from build123d import *

# Parameters (mm, degrees)
BOSS_EXTRUDE1_DEPTH      = 50.8
BOSS_EXTRUDE1_DEPTH_BACK = 38.1
SKETCH1_W                = 381
SKETCH1_H                = 12.7
SKETCH3_W                = 12.7
SKETCH3_H                = 44.45
CUT_EXTRUDE1_DEPTH       = 2664.230012597
CAVITY1_START            = 52.3
CAVITY1_OUTLINE_R        = 12.7
CAVITY1_DEPTH            = 12.7


# Read off the part's stored shape, not the designer's step: Cavity1
with BuildPart() as part:
    # Sketch1 → Boss-Extrude1 (new, two sides: drawn at the far end of the back side and taken through both)
    with BuildSketch(Plane.XY.offset(287.7).offset(-BOSS_EXTRUDE1_DEPTH_BACK)):
        with Locations((2451.1, 58.65)):
            Rectangle(SKETCH1_W, SKETCH1_H)
    extrude(amount=BOSS_EXTRUDE1_DEPTH + BOSS_EXTRUDE1_DEPTH_BACK)

    # Sketch3 → Cut-Extrude1 (cut, through all)
    with BuildSketch(Plane(origin=(0, 65, 0), x_dir=(1, 0, 0), z_dir=(0, 1, 0))):
        with Locations((2470.15, -271.825)):
            Rectangle(SKETCH3_W, SKETCH3_H)
    extrude(amount=-CUT_EXTRUDE1_DEPTH, mode=Mode.SUBTRACT)

    # Cavity1 outline → Cavity1 (cut)
    with BuildSketch(Plane(origin=(0, 0, 0), x_dir=(1, 0, 0), z_dir=(0, 1, 0)).offset(CAVITY1_START)):
        with Locations((2300, -275)):
            Circle(CAVITY1_OUTLINE_R)
        with Locations((2600, -275)):
            Circle(CAVITY1_OUTLINE_R)
    extrude(amount=CAVITY1_DEPTH, mode=Mode.SUBTRACT)


solid = part.part
Can you work these out from the model? Positions are in its coordinate system, mm. A direction names the side the tool comes from. Give positions to 0.01 mm unless a question says otherwise; leave off trailing zeros. Order: outer loops, then holes, each group sorted by start corner. A loop starts at its lowest first (then second) coordinate and runs counter-clockwise, first axis right, second up. Notation, with made-up numbers: M 20.25,88.25 L 43.25,88.25 A26 ccw 43.25,108.25 Z; hole C 33,-9 d5. An arc over 180 degrees is marked long. One line per item, written item: value.
Item 1: If we section it at C-C on y = 60.5: Write out the boundary of the cut face in (x, z).
Verdict:
outline: M 2260.6,249.6 L 2463.8,249.6 L 2463.8,294.05 L 2476.5,294.05 L 2476.5,249.6 L 2641.6,249.6 L 2641.6,338.5 L 2260.6,338.5 Z; hole C 2300,275 d25.4; hole C 2600,275 d25.4
Item 2: For faces 5 (the face through (2361, 59, 249.6)), 6 (the face through (2470, 59, 294.05)), which set-ups out of +Z, -Z, +X, -X, +Y, -Y let a thin tool reach every point of the face, with its end or its side?
Verdict:
face 5: -Z, +X, -X, +Y, -Y
face 6: -Z, +Y, -Y
Item 3: For pin 1 (23 mm diameter, centred on x = 2300, z = 275, fed in from -Y), with a flat end and sliding along its axis, tell me the tip position at first contact or that it passes through.
Verdict:
pin 1: through
Item 4: If we section it at B-B on x = 2300: Write out the boundary of the cut face in (y, z), and give its area (3 significant figures).
Verdict:
outline: M 52.3,249.6 L 65,249.6 L 65,262.3 L 52.3,262.3 Z; M 52.3,287.7 L 65,287.7 L 65,338.5 L 52.3,338.5 Z
area: 806 mm2
Item 5: Please list where these lines run through material, in increasing order: line 1 (X direction, y = 57.5, z = 275); line 2 (Z direction, x = 2300, y = 57); line 3 (X direction, y = 59, z = 268.5).
Verdict:
line 1: 2260.6 to 2287.3, 2312.7 to 2463.8, 2476.5 to 2587.3, 2612.7 to 2641.6
line 2: 249.6 to 262.3, 287.7 to 338.5
line 3: 2260.6 to 2289.09, 2310.91 to 2463.8, 2476.5 to 2589.09, 2610.91 to 2641.6
Item 6: If we section it at A-A on z = 275: Write out the boundary of the cut face in (x, y).
Verdict:
outline: M 2260.6,52.3 L 2287.3,52.3 L 2287.3,65 L 2260.6,65 Z; M 2312.7,52.3 L 2463.8,52.3 L 2463.8,65 L 2312.7,65 Z; M 2476.5,52.3 L 2587.3,52.3 L 2587.3,65 L 2476.5,65 Z; M 2612.7,52.3 L 2641.6,52.3 L 2641.6,65 L 2612.7,65 Z
Item 7: If we mould it in two halves opening along X, with no side actions, what happens to faces 1 (the face through (2448, 59, 338.5)), 2 (the face through (2641.6, 59, 293)), 3 (the face through (2587.312, 58.561, 274.442)), 4 (the face through (2463.8, 59, 272))? For each: pulls with the +X half, pulls with the -X half, needs draft (parallel to the pull), parting line crosses it, or undercut.
Verdict:
face 1: needs draft
face 2: pulls with the +X half
face 3: undercut
face 4: undercut
